Can you work these out from the model? Positions are in its coordinate system, mm. Face numbers are marked on the shaded views. A direction names the side the tool comes from. Round coordinates to 2 decimals unless told otherwise and drop trailing zeros. Loops run counter-clockwise (first coordinate to the right, second up) from the corner with the lowest first, then second, coordinate; pieces in that order, holes last.
(1) If I drill on line 1 along Y through (x, z) = (0, 1.45) (3 decimals); line 2 along Z through (x, y) = (2.5, 5.25); line 3 along X through (y, z) = (-4.75, 19.25), over which ranges is the centre line in solid material (lowest first)?
(2) I want a section at C-C on x = -68. Write out the boundary of the cut face in (y, z) (3 decimals), plus the area to 4 significant figures.
(3) Which directions (+Z, -Z, +X, -X, +Y, -Y) give clear straight access to the entire face, cutting with the end or side of a thin tool? Please do the marked faces 1, 2, 3, 4 and 5.
(4) I want a section at B-B on z = 20.5. Write out the boundary of the cut face in (x, y) (3 decimals), plus the area to 3 significant figures.
(5) I want a section at A-A on y = 0. Write out the boundary of the cut face in (x, z) (3 decimals), plus the area to 3 significant figures.
(6) Thinking about a two-plate mould opening in Y: for the marked faces 6, 7 and 8, which applies, released by +Y, released by -Y, zero draft, split by the parting line, or undercut?
(7) Will these pins go through, and if not, where does the flat tip stop? pin 1 Ø5.5 at (y, z) = (5.5, 22) entering from +X; pin 2 Ø4 at (x, y) = (-52.5, 5.5) entering from +Z; pin 3 Ø4 at (y, z) = (-3.5, 15) entering from +X.
(8) I want a section at D-D on y = 7.5. Write out the boundary of the cut face in (x, z).
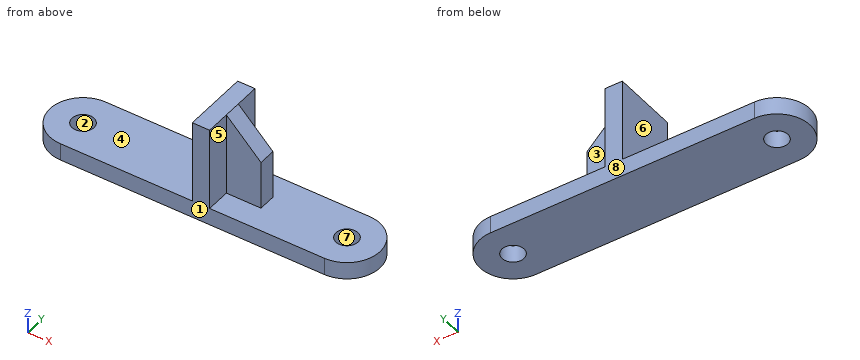
Autodesk Inventor part; units mm, degrees
ref_plane "YZ Plane" through (0, 0, 0) normal (1, 0, 0) x (0, 1, 0)
ref_plane "XZ Plane" through (0, 0, 0) normal (0, 1, 0) x (-1, 0, 0)
ref_plane "XY Plane" through (0, 0, 0) normal (0, 0, 1) x (1, 0, 0)
sketch "Sketch1" plane through (0, 0, 0) normal (0, 0, 1) x (1, 0, 0)
  circle A0 centre (0, 0) radius 3.175
  circle A1 centre (-76.2, 0) radius 3.175
  arc A2 (-76.2, 9.525) -> (-76.2, -9.525) centre (-76.2, 0) ccw
  arc A3 (0, -9.525) -> (0, 9.525) centre (0, 0) ccw
  line L0 (-76.2, 9.525) -> (0, 9.525)
  line L1 (-76.2, -9.525) -> (0, -9.525)
  dimension "d0" = 6.35
  dimension "d1" = 6.35
  dimension "d2" = 76.2
  dimension "d3" = 6.35
  dimension "d4" = 6.35
extrude "Extrusion1" add sketch "Sketch1" along normal blind 5
sketch "Sketch2" plane through (0, 0, 5) normal (0, 0, 1) x (1, 0, 0)
  line L0 (0, 9.525) -> (-76.2, 9.525)
  line L1 (-76.2, -9.525) -> (0, -9.525)
  line L2 (-38.1, 9.525) -> (-33.1, 9.525)
  line L3 (-33.1, 9.525) -> (-33.1, -9.525)
  line L4 (-33.1, -9.525) -> (-38.1, -9.525)
  line L5 (-38.1, -9.525) -> (-38.1, 9.525)
  line L6 (-33.1, 2.5) -> (-23.1, 2.5)
  line L7 (-23.1, 2.5) -> (-23.1, -2.5)
  line L8 (-23.1, -2.5) -> (-33.1, -2.5)
  line L9 (-33.1, -2.5) -> (-33.1, 2.5)
  line L10 (-23.1, 0) -> (-38.1, 0) construction
  point P0 (0, 0)
  dimension "d7" = 5
  dimension "d8" = 10
  dimension "d9" = 5
extrude "Extrusion2" add sketch "Sketch2" along normal blind 24
chamfer "Chamfer1" distance 10 angle 45 1 edges at (-23.1, 0, 29)
properties part number "Y Axis Limit Switch Trigger"
Filled sheet:
1. line 1: y = -9.525 to -3.175, 3.175 to 9.525
1. line 2: z = 0 to 5
1. line 3: x = -38.1 to -33.1
2. outline: (-9.525, 0) - (9.525, 0) - (9.525, 5) - (-9.525, 5) - close
2. area: 95.25 mm2
3. face 1: +Z, -Z, +X, -X, -Y
3. face 2: +Z, -Z
3. face 3: +Z, +X, +Y
3. face 4: +Z, -X, +Y, -Y
3. face 5: +Z, +X, -Y
4. outline: (-38.1, -9.525) - (-33.1, -9.525) - (-33.1, -2.5) - (-24.6, -2.5) - (-24.6, 2.5) - (-33.1, 2.5) - (-33.1, 9.525) - (-38.1, 9.525) - close
4. area: 138 mm2
5. outline: (-85.725, 0) - (-79.375, 0) - (-79.375, 5) - (-85.725, 5) - close; (-73.025, 0) - (-3.175, 0) - (-3.175, 5) - (-23.1, 5) - (-23.1, 19) - (-33.1, 29) - (-38.1, 29) - (-38.1, 5) - (-73.025, 5) - close; (3.175, 0) - (9.525, 0) - (9.525, 5) - (3.175, 5) - close
5. area: 723 mm2
6. face 6: zero draft
6. face 7: undercut
6. face 8: released by +Y
7. pin 1: stops at x = -33.1
7. pin 2: stops at z = 5
7. pin 3: stops at x = -23.1
8. outline: (-82.07, 0) - (5.87, 0) - (5.87, 5) - (-33.1, 5) - (-33.1, 29) - (-38.1, 29) - (-38.1, 5) - (-82.07, 5) - close
